For this review, take the finished solid that the model builds, in its own axes (mm). A direction names the side the tool comes from. Give positions to 0.01 mm unless a question says otherwise; leave off trailing zeros. Loops run counter-clockwise (first coordinate to the right, second up) from the corner with the lowest first, then second, coordinate; pieces in that order, holes last. Notation, with made-up numbers: (62, -2) -> (77, -2) arc R17 cw to (77, 10) -> close; hole circle Ø4 at (-29.5, -27). An arc over 180 degrees is marked (long way). One line per question, with ' | ' between items. Start each with the question number.
(1) Consider section B-B (y = 8.5). Write out the cut boundary in (x, z).
(2) Draft analysis for pull direction Y (two halves, no side actions). For faces 1 (the flat face through (-73, 76.5, 4)), 2 (the flat face through (-1, 40, 63.5)), 3 (the flat face through (-40, 79, 63.5)), 4 (the flat face through (-43, 0, 8)), state which applies: +Y half, -Y half, draft (parallel to the pull), parting line (faces both ways), or undercut.
(3) Wall thickness on probe 1 along X at (y, z) = (7, 39.5); probe 2 along Y at (x, z) = (-11, 23); probe 3 along Y at (x, z) = (-49.5, 25.5): over which ranges is each line inside the solid? List them lowest first.
(4) Tool access review of faces 5 (the flat face through (-67.5, 1, 36)), 6 (the flat face through (-79, 40, 63.5)), 7 (the flat face through (-12.5, 40, 64)), 8 (the flat face through (-40, 78, 36)), 9 (the flat face through (-77, 4, 6.6)): name each direction out of +Z, -Z, +X, -X, +Y, -Y from which nothing blocks a thin tool from reaching the whole face with its end or side.
(5) Consider section C-C (x = -8.5). Write out the cut boundary in (y, z), and give its area (3 significant figures).
(6) Consider section A-A (z = 55). Write out the cut boundary in (x, y), and give its area (3 significant figures).
(7) Insertion check: P1, Ø2, axis at x = -79, y = 45, coming from the -Z side; P2, Ø5, axis at x = -25.5, y = 60, coming from the +Z side; P3, Ø10, axis at y = 34.5, z = 26.5, coming from the -X side; P4, Ø18, axis at x = -54, z = 43, coming from the +Y side. Each pin has a flat end and moves straight along its axis. Give the tip position at first contact, or say it passes through.
(8) Consider section D-D (y = 65.5). Write out the cut boundary in (x, z).
Autodesk Inventor part; units mm, degrees
ref_plane "YZ Plane" through (0, 0, 0) normal (1, 0, 0) x (0, 1, 0)
ref_plane "XZ Plane" through (0, 0, 0) normal (0, 1, 0) x (-1, 0, 0)
ref_plane "XY Plane" through (0, 0, 0) normal (0, 0, 1) x (1, 0, 0)
sketch "Sketch7" plane through (0, 0, 0) normal (0, 0, 1) x (1, 0, 0)
  line L0 (0, 0) -> (-80, 0)
  line L1 (-80, 0) -> (-80, 80)
  line L2 (-80, 80) -> (0, 80)
  line L3 (0, 80) -> (0, 0)
  line L4 (-75, 75) -> (-5, 75)
  line L5 (-5, 75) -> (-5, 5)
  line L6 (-5, 5) -> (-75, 5)
  line L7 (-75, 5) -> (-75, 75)
  dimension "d54" = 80
  dimension "d55" = 80
  dimension "d56" = 70
  dimension "d57" = 70
extrude "Extrusion10" add sketch "Sketch7" along normal blind 60
sketch "Sketch8" plane through (0, 0, 60) normal (0, 0, 1) x (1, 0, 0)
  line L0 (0, 0) -> (0, 80)
  line L1 (0, 0) -> (-80, 0)
  line L2 (-80, 0) -> (-80, 80)
  line L3 (-80, 80) -> (0, 80)
  line L4 (0, 80) -> (0, 0)
  dimension "d60" = 80
  dimension "d61" = 80
extrude "Extrusion11" add sketch "Sketch8" along normal blind 5
sketch "Sketch9" plane through (0, 0, 65) normal (0, 0, 1) x (1, 0, 0)
  line L0 (-12.5, 12.5) -> (-67.5, 12.5)
  line L1 (-67.5, 12.5) -> (-67.5, 67.5)
  line L2 (-67.5, 67.5) -> (-12.5, 67.5)
  line L3 (-12.5, 67.5) -> (-12.5, 12.5)
  point P0 (0, 0)
  dimension "d64" = 55
  dimension "d65" = 55
extrude "Extrusion12" cut sketch "Sketch9" against normal blind 2
sketch "Sketch10" plane through (0, 0, 0) normal (1, 0, 0) x (0, 0, -1)
  line L0 (-63.5, 12.5) -> (-8.5, 12.5)
  line L1 (-8.5, 12.5) -> (-8.5, 67.5)
  line L2 (-8.5, 67.5) -> (-63.5, 67.5)
  line L3 (-63.5, 67.5) -> (-63.5, 12.5)
  point P0 (0, 0)
  dimension "d68" = 55
  dimension "d69" = 55
extrude "Extrusion13" cut sketch "Sketch10" against normal blind 2
sketch "Sketch11" plane through (-80, 80, 0) normal (0, 1, 0) x (1, 0, 0)
  line L0 (12.5, -63.5) -> (67.5, -63.5)
  line L1 (67.5, -63.5) -> (67.5, -8.5)
  line L2 (67.5, -8.5) -> (12.5, -8.5)
  line L3 (12.5, -8.5) -> (12.5, -63.5)
  point P0 (80, 0)
  dimension "d72" = 55
  dimension "d73" = 55
sketch "Sketch12" plane through (-80, 0, 0) normal (-1, 0, 0) x (0, 0, 1)
  line L0 (63.5, 12.5) -> (8.5, 12.5)
  line L1 (8.5, 12.5) -> (8.5, 67.5)
  line L2 (8.5, 67.5) -> (63.5, 67.5)
  line L3 (63.5, 67.5) -> (63.5, 12.5)
  point P0 (0, 0)
  dimension "d74" = 55
  dimension "d75" = 55
sketch "Sketch13" plane through (-80, 0, 0) normal (0, -1, 0) x (1, 0, 0)
  line L0 (12.5, 63.5) -> (67.5, 63.5)
  line L1 (67.5, 63.5) -> (67.5, 8.5)
  line L2 (67.5, 8.5) -> (12.5, 8.5)
  line L3 (12.5, 8.5) -> (12.5, 63.5)
  point P0 (80, 0)
  dimension "d76" = 55
  dimension "d77" = 55
extrude "Extrusion14" cut sketch "Sketch11" against normal blind 2
extrude "Extrusion15" cut sketch "Sketch12" against normal blind 2
extrude "Extrusion16" cut sketch "Sketch13" against normal blind 2
sketch "Sketch14" plane through (-80, 80, 0) normal (0, 1, 0) x (1, 0, 0)
  line L0 (79, -1) -> (68.4, -1)
  line L1 (68.4, -1) -> (68.4, -6.6)
  line L2 (68.4, -6.6) -> (79, -6.6)
  line L3 (79, -6.6) -> (79, -1)
  line L4 (1, -1) -> (11.6, -1)
  line L5 (11.6, -1) -> (11.6, -6.6)
  line L6 (11.6, -6.6) -> (1, -6.6)
  line L7 (1, -6.6) -> (1, -1)
  point P0 (80, 0)
  dimension "d84" = 10.6
  dimension "d85" = 5.6
  dimension "d86" = 10.6
  dimension "d87" = 5.6
extrude "Extrusion17" cut sketch "Sketch14" against normal blind 3.5
sketch "Sketch15" plane through (-80, 0, 0) normal (-1, 0, 0) x (0, 0, 1)
  line L0 (1, 1) -> (6.6, 1)
  line L1 (6.6, 1) -> (6.6, 11.6)
  line L2 (6.6, 11.6) -> (1, 11.6)
  line L3 (1, 11.6) -> (1, 1)
  line L4 (1, 79) -> (6.6, 79)
  line L5 (6.6, 79) -> (6.6, 68.4)
  line L6 (6.6, 68.4) -> (1, 68.4)
  line L7 (1, 68.4) -> (1, 79)
  point P0 (0, 0)
  dimension "d90" = 5.6
  dimension "d91" = 10.6
  dimension "d92" = 5.6
  dimension "d93" = 10.6
sketch "Sketch16" plane through (-80, 0, 0) normal (0, -1, 0) x (1, 0, 0)
  line L0 (1, 1) -> (11.6, 1)
  line L1 (11.6, 1) -> (11.6, 6.6)
  line L2 (11.6, 6.6) -> (1, 6.6)
  line L3 (1, 6.6) -> (1, 1)
  line L4 (79, 1) -> (68.4, 1)
  line L5 (68.4, 1) -> (68.4, 6.6)
  line L6 (68.4, 6.6) -> (79, 6.6)
  line L7 (79, 6.6) -> (79, 1)
  point P0 (80, 0)
  dimension "d94" = 10.6
  dimension "d95" = 5.6
  dimension "d96" = 10.6
  dimension "d97" = 5.6
sketch "Sketch17" plane through (0, 0, 0) normal (1, 0, 0) x (0, 0, -1)
  line L0 (-1, 1) -> (-6.6, 1)
  line L1 (-6.6, 1) -> (-6.6, 11.6)
  line L2 (-6.6, 11.6) -> (-1, 11.6)
  line L3 (-1, 11.6) -> (-1, 1)
  line L4 (-1, 79) -> (-6.6, 79)
  line L5 (-6.6, 79) -> (-6.6, 68.4)
  line L6 (-6.6, 68.4) -> (-1, 68.4)
  line L7 (-1, 68.4) -> (-1, 79)
  point P0 (0, 0)
  dimension "d98" = 5.6
  dimension "d99" = 10.6
  dimension "d100" = 5.6
  dimension "d101" = 10.6
extrude "Extrusion18" cut sketch "Sketch17" against normal blind 3.5
extrude "Extrusion19" cut sketch "Sketch16" against normal blind 3.5
extrude "Extrusion20" cut sketch "Sketch15" against normal blind 3.5
properties part number "Circle_TestFit_V1"
A:
1) outline: (-80, 0) -> (-75, 0) -> (-75, 60) -> (-5, 60) -> (-5, 0) -> (0, 0) -> (0, 1) -> (-3.5, 1) -> (-3.5, 6.6) -> (0, 6.6) -> (0, 65) -> (-80, 65) -> (-80, 6.6) -> (-76.5, 6.6) -> (-76.5, 1) -> (-80, 1) -> close
2) face 1: +Y half | face 2: undercut | face 3: draft | face 4: -Y half
3) probe 1: x = -80 to -75, -5 to 0 | probe 2: y = 0 to 5, 75 to 80 | probe 3: y = 2 to 5, 75 to 78
4) face 5: -Y | face 6: -X | face 7: +Z | face 8: +Y | face 9: none
5) outline: (0, 0) -> (5, 0) -> (5, 60) -> (75, 60) -> (75, 0) -> (80, 0) -> (80, 1) -> (76.5, 1) -> (76.5, 6.6) -> (80, 6.6) -> (80, 65) -> (0, 65) -> (0, 6.6) -> (3.5, 6.6) -> (3.5, 1) -> (0, 1) -> close | area: 961 mm^2
6) outline: (-80, 0) -> (-67.5, 0) -> (-67.5, 2) -> (-12.5, 2) -> (-12.5, 0) -> (0, 0) -> (0, 12.5) -> (-2, 12.5) -> (-2, 67.5) -> (0, 67.5) -> (0, 80) -> (-12.5, 80) -> (-12.5, 78) -> (-67.5, 78) -> (-67.5, 80) -> (-80, 80) -> (-80, 67.5) -> (-78, 67.5) -> (-78, 12.5) -> (-80, 12.5) -> close; hole (-75, 5) -> (-5, 5) -> (-5, 75) -> (-75, 75) -> close | area: 1,060 mm^2
7) P1: stops at z = 0 | P2: stops at z = 63 | P3: stops at x = -78 | P4: stops at y = 78
8) outline: (-80, 0) -> (-75, 0) -> (-75, 60) -> (-5, 60) -> (-5, 0) -> (0, 0) -> (0, 8.5) -> (-2, 8.5) -> (-2, 63.5) -> (0, 63.5) -> (0, 65) -> (-12.5, 65) -> (-12.5, 63) -> (-67.5, 63) -> (-67.5, 65) -> (-80, 65) -> (-80, 63.5) -> (-78, 63.5) -> (-78, 8.5) -> (-80, 8.5) -> close
